Geometry: final body of the model. Coordinates: model frame, mm. A direction names the side the tool comes from. Give positions to 0.01 mm unless a question says otherwise; leave off trailing zeros. Write each loop counter-clockwise with the first axis right and the second up, starting at its lowest first coordinate (ties: lowest second). Pieces come first, ordered by that corner, then holes. Notation, with made-up numbers: (31, 34.25) -> (51, 34.25) arc R27 ccw to (51, 66.25) -> close; hole circle Ø1 at (-4.5, 20.5). An arc over 180 degrees is marked (long way). Answer as a JSON object with one key per item and string values.
from build123d import *

# Parameters (mm, degrees)
F3_W     = 101.6
F3_H     = 76.2
F3_W_2   = 76.2
F3_H_2   = 101.6
F4_DEPTH = 6.35


with BuildPart() as f1:
    # F0 (on Right) → F1 (revolve)
    with BuildSketch(Plane.YZ):
        Polygon((-581.025, 1524), (-584.2, 1524), (-584.2, 0), (-78.445064, -505.754936), (-76.2, -503.509872), (-581.025, 1.315128), align=None)
    revolve(axis=Axis((0, 0, 0), (0, 0, -1)))

    # F3 (on offset) → F4 (join)
    with BuildSketch(Plane.XY.offset(1092.2)):
        with Locations((0, 620.087113)):
            Rectangle(F3_W, F3_H)
        with Locations((-620.087113, 0)):
            Rectangle(F3_W_2, F3_H_2)
        with Locations((0, -620.087113)):
            Rectangle(F3_W, F3_H)
        with Locations((620.087113, 0)):
            Rectangle(F3_W_2, F3_H_2)
    extrude(amount=F4_DEPTH)


solid = f1.part
Q1. Cut plane A-A (x = 0). Return the cut outline in (y, z) (3 decimals).
Values:
{"outline": "(-658.187, 1092.2) -> (-584.2, 1092.2) -> (-584.2, 0) -> (-78.445, -505.755) -> (-76.2, -503.51) -> (-581.025, 1.315) -> (-581.025, 1524) -> (-584.2, 1524) -> (-584.2, 1098.55) -> (-658.187, 1098.55) -> close; (76.2, -503.51) -> (78.445, -505.755) -> (584.2, 0) -> (584.2, 1092.2) -> (658.187, 1092.2) -> (658.187, 1098.55) -> (584.2, 1098.55) -> (584.2, 1524) -> (581.025, 1524) -> (581.025, 1.315) -> close"}
Q2. Material intervals for L1, parallel to X at y = 0, z = 1063.5 (3 decimals); L2, parallel to Y at x = 13.5, z = 641.5, sorted ascending. Write a range as from..to.
Values:
{"L1": "-584.2..-581.025, 581.025..584.2", "L2": "-584.04..-580.87, 580.87..584.04"}
Q3. Mould query, pull axis Y, two halves, no side actions, for faces 1 (the flat face through (620, 1, 1098.55)), 2 (the conical face through (-7.21, 163.71, -415.84)), 3 (the conical face through (-47.82, -151.85, -425)). Classes: pulls with the +Y half, pulls with the -Y half, needs draft (parallel to the pull), parting line crosses it, or undercut.
Values:
{"face 1": "needs draft", "face 2": "undercut", "face 3": "parting line crosses it"}
Q4. Cut plane D-D (z = 1126). Return the cut outline in (x, y) (3 decimals).
Values:
{"outline": "circle Ø1168.4 at (0, 0); hole circle Ø1162.05 at (0, 0)"}
Q5. Cut plane C-C (z = -140.5). Return the cut outline in (x, y), and give its area (3 significant figures).
Values:
{"outline": "circle Ø887.4 at (0, 0); hole circle Ø878.42 at (0, 0)", "area": "12,500 mm²"}
Q6. First-contact query: P1, Ø3, axis at y = 604.5, z = 1096, coming from the +X side; P2, Ø23, axis at x = -20.5, y = 636, coming from the +Z side; P3, Ø1.9, axis at x = 634.5, z = 1094.5, coming from the -Y side. Flat tips, straight axial feed; report the tip coordinate or a pass-through.
Values:
{"P1": "x = 50.8", "P2": "z = 1098.55", "P3": "y = -50.8"}
Q7. Set-up query: faces 4 (the cylindrical face through (567.2, 126, 773.3)), 5 (the conical face through (-22.921, -72.785, -503.619)). Return all of +Z, -Z, +X, -X, +Y, -Y with unobstructed straight access to the full face (end or side cutting, diameter ignored); none if empty.
Values:
{"face 4": "+Z", "face 5": "-Z"}
